For this review, take the finished solid that the model builds, in its own axes (mm). Face numbers are marked on the shaded views. A direction names the side the tool comes from. Round coordinates to 2 decimals unless told otherwise and drop trailing zeros. Write each loop counter-clockwise with the first axis right and the second up, starting at its lowest first coordinate (ties: lowest second). Pieces come first, ordered by that corner, then holes. Notation, with made-up numbers: (18, -12.75) -> (26, -12.75) arc R5 cw to (26, -4.75) -> close; hole circle Ø3 at (48, 88.25). An arc over 180 degrees is marked (long way). Write each question's results on one line, items separated by ' | '. Start each with the question number.
Item 1: Tool access review of the marked faces 1, 2 and 3: name each direction out of +Z, -Z, +X, -X, +Y, -Y from which nothing blocks a thin tool from reaching the whole face with its end or side.
Item 2: Add section B-B (x = 23.5). State the section outline as (y, z) points.
Item 3: Clearance check with flat-ended pins moving along their axes: pin 1 (3 mm diameter, centred on y = 13.5, z = -8, fed in from -X); pin 2 (1.1 mm diameter, centred on x = 37.5, z = -7.5, fed in from -Y); pin 3 (5 mm diameter, centred on y = 13.5, z = 6.5, fed in from +X). State where each tip first meets the part, or that it passes through.
Item 4: Add section D-D (x = 17). State the section outline as (y, z) points, plus the area to 3 significant figures.
Item 5: The part is to be moulded in two halves that separate along Z. For the marked faces 4, 5, 6 and 7, say which applies: +Z half, -Z half, draft (parallel to the pull), parting line (faces both ways), or undercut.
Item 6: Add section A-A (y = 8.25). State the section outline as (x, z) points.
Item 7: To check wall thickness, follow line 1 along Z through (x, y) = (23, 12.75); line 2 along Y through (x, z) = (6.5, 1.5); line 3 along X through (y, z) = (2, 7.5). State the ranges of each line that lie inside material, in increasing order.
Item 8: Add section C-C (y = 1). State the section outline as (x, z) points.
from build123d import *

# Parameters (mm, degrees)
SKETCH_1_W           = 40
SKETCH_1_H           = 20
EXTRUDE_1_DEPTH      = 20
SKETCH_2_W           = 8
SKETCH_2_H           = 4
EXTRUDE_2_DEPTH      = 16
SKETCH_4_W           = 12
SKETCH_4_H           = 18.32487869
CUT_EXTRUDE_2_DEPTH  = 41
SKETCH_7_W           = 12
SKETCH_7_H           = 4
CUT_EXTRUDE_4_DEPTH  = 20
SKETCH_5_R           = 1
EXTRUDE_3_DEPTH      = 10
SKETCH_6_W           = 8
SKETCH_6_H           = 25.038569191
CUT_EXTRUDE_3_DEPTH  = 10
CUT_EXTRUDE_8_DEPTH  = 20
SKETCH_13_R          = 1
EXTRUDE_5_DEPTH      = 8
CUT_EXTRUDE_10_DEPTH = 20
SKETCH_16_R          = 1
EXTRUDE_12_DEPTH     = 5
SKETCH_17_R          = 1
EXTRUDE_13_DEPTH     = 5


with BuildPart() as part:
    # 草图1 → 凸台-拉伸1 (new body)
    with BuildSketch(Plane(origin=(0, 0, 0), x_dir=(1, 0, 0), z_dir=(0, 1, 0))):
        with Locations((18, 0)):
            Rectangle(SKETCH_1_W, SKETCH_1_H)
    extrude(amount=EXTRUDE_1_DEPTH)

    # 草图2 → 凸台-拉伸2 (add)
    with BuildSketch(Plane.ZY.offset(2)):
        with Locations((0, 2)):
            Rectangle(SKETCH_2_W, SKETCH_2_H)
    extrude(amount=EXTRUDE_2_DEPTH)

    # 草图4 → 切除-拉伸2 (cut, through all)
    with BuildSketch(Plane.ZY.offset(2)):
        with Locations((0, 13.162439345)):
            Rectangle(SKETCH_4_W, SKETCH_4_H)
    extrude(amount=-CUT_EXTRUDE_2_DEPTH, mode=Mode.SUBTRACT)

    # 草图7 → 切除-拉伸4 (cut)
    with BuildSketch(Plane(origin=(38, 0, 0), x_dir=(0, 0, -1), z_dir=(1, 0, 0))):
        with Locations((0, 2)):
            Rectangle(SKETCH_7_W, SKETCH_7_H)
    extrude(amount=-CUT_EXTRUDE_4_DEPTH, mode=Mode.SUBTRACT)

    # 草图5 → 凸台-拉伸3 (add, symmetric)
    with BuildSketch(Plane.XY):
        with Locations((38, 19)):
            Circle(SKETCH_5_R)
        with Locations((38, 1)):
            Circle(SKETCH_5_R)
    extrude(amount=EXTRUDE_3_DEPTH, both=True)

    # 草图6 → 切除-拉伸3 (cut, symmetric)
    with BuildSketch(Plane(origin=(38, 0, 0), x_dir=(0, 0, -1), z_dir=(1, 0, 0))):
        with Locations((0, 10.475013396)):
            Rectangle(SKETCH_6_W, SKETCH_6_H)
    extrude(amount=CUT_EXTRUDE_3_DEPTH, both=True, mode=Mode.SUBTRACT)

    # 草图12 → 切除-拉伸8 (cut)
    with BuildSketch(Plane.XY.offset(4)):
        with BuildLine():
            Line((-5, 2), (-18.474771325, 2))
            Line((-18.474771325, 2), (-18.474771325, 0))
            Line((-18.474771325, 0), (-5, 0))
            ThreePointArc((-5, 0), (-6, 1), (-5, 2))
        make_face()
    extrude(amount=-CUT_EXTRUDE_8_DEPTH, mode=Mode.SUBTRACT)

    # 草图13 → 凸台-拉伸5 (add)
    with BuildSketch(Plane.XY.offset(4)):
        with Locations((-18, 3)):
            Circle(SKETCH_13_R)
    extrude(amount=-EXTRUDE_5_DEPTH)

    # 草图15 → 切除-拉伸10 (cut)
    with BuildSketch(Plane.XY.offset(10)):
        Polygon((19, 0), (39.887994795, 0), (38, 18), (37, 18), align=None)
    extrude(amount=-CUT_EXTRUDE_10_DEPTH, mode=Mode.SUBTRACT)

    # 草图16 → 凸台-拉伸12 (add)
    with BuildSketch(Plane.XY.offset(10)):
        with Locations((20, 1)):
            Circle(SKETCH_16_R)
    extrude(amount=-EXTRUDE_12_DEPTH)

    # 草图17 → 凸台-拉伸13 (add)
    with BuildSketch(Plane(origin=(0, 0, -10), x_dir=(-1, 0, 0), z_dir=(0, 0, -1))):
        with Locations((-20, 1)):
            Circle(SKETCH_17_R)
    extrude(amount=-EXTRUDE_13_DEPTH)


solid = part.part
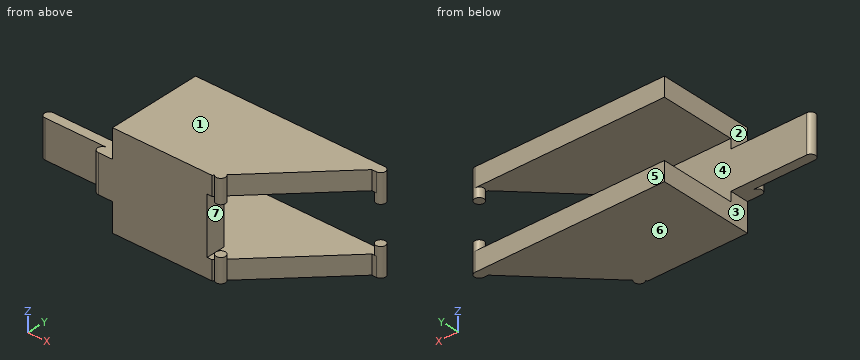
Responses:
1) face 1: +Z, +X, -X, +Y, -Y | face 2: +Z, -X, +Y, -Y | face 3: -Z, -X, +Y, -Y
2) outline: (4.5, -10) -> (20, -10) -> (20, -6) -> (4.5, -6) -> close; (4.5, 6) -> (20, 6) -> (20, 10) -> (4.5, 10) -> close
3) pin 1: stops at x = -2 | pin 2: stops at y = 17.95 | pin 3: stops at x = 35
4) outline: (0, -10) -> (20, -10) -> (20, -6) -> (4, -6) -> (4, 6) -> (20, 6) -> (20, 10) -> (0, 10) -> close | area: 208 mm^2
5) face 4: undercut | face 5: draft | face 6: -Z half | face 7: undercut
6) outline: (-2, -10) -> (27.25, -10) -> (27.25, -6) -> (-2, -6) -> close; (-2, 6) -> (27.25, 6) -> (27.25, 10) -> (-2, 10) -> close
7) line 1: z = -10 to -6, 6 to 10 | line 2: y = 0 to 4 | line 3: x = -2 to 21
8) outline: (-6, -4) -> (-2, -4) -> (-2, -10) -> (21, -10) -> (21, -5) -> (19, -5) -> (19, -6) -> (18, -6) -> (18, 6) -> (19, 6) -> (19, 5) -> (21, 5) -> (21, 10) -> (-2, 10) -> (-2, 4) -> (-6, 4) -> close
